CAD build for the part. Positions are in the model's coordinates, mm. Give positions to 0.01 mm unless a question says otherwise; leave off trailing zeros. Write each loop counter-clockwise with the first axis right and the second up, starting at its lowest first coordinate (ties: lowest second). Pieces come first, ordered by that corner, then holes. Notation, with made-up numbers: (24, 57.25) - (29, 57.25) arc R15 cw to (29, 68.25) - close; hole circle Ø7 at (31.5, 51.25). An arc over 180 degrees is marked (long way). Put each result on its own line as item: value. Start each with the question number.
1. Mould opens along X. For faces 1 (the cylindrical face through (-9.162, 40.474, 298.893)), 2 (the flat face through (38.538, 18, 148)), 3 (the cylindrical face through (-0.702, 40.994, 147.9)), 4 (the flat face through (-38.538, 18, 148)) say: +X half, -X half, draft (parallel to the pull), parting line (faces both ways), or undercut.
2. Drop flat-ended pins along their axis: pin 1 (3.5 mm diameter, centred on x = 0, z = 41, fed in from -Y); pin 2 (12 mm diameter, centred on x = 7, z = 53.5, fed in from -Y); pin 3 (8 mm diameter, centred on y = 36.5, z = 242.5, fed in from -X); pin 4 (3 mm diameter, centred on x = 0, z = 10, fed in from +Y). Give the stop position or say it passes through.
3. Wall check: line 1 (X direction, y = 41, z = 10); line 2 (X direction, y = 33, z = 35); line 3 (Y direction, x = 1.5, z = 92). Give the ranges that are in metal, low to high.
4. Cut at B-B on z = 134. List the corners of the cut face in (x, y), and give its area (3 significant figures).
5. Cut at C-C on x = 23.5. List the corners of the cut face in (y, z), and give its area (3 significant figures).
6. Cut at A-A on y = 26. List the corners of the cut face in (x, z), and give its area (3 significant figures).
from build123d import *

# Parameters (mm, degrees)
BOSS_EXTRU_1_DEPTH                   = 300
ENL_V_MAT_EXTRU_1_DEPTH              = 45.5
D_GAGEMENT_M21_D                     = 3.1
D_GAGEMENT_M21_CSINK_D               = 6
D_GAGEMENT_M21_CSINK_ANGLE           = 120
R_P_TITION_LIN_AIRE1_COUNT           = 2
R_P_TITION_LIN_AIRE1_PITCH           = 31
D_GAGEMENT_M41_D                     = 3.1
D_GAGEMENT_M41_DEPTH                 = 30
D_GAGEMENT_M41_CSINK_D               = 5
D_GAGEMENT_M41_CSINK_ANGLE           = 90
D_GAGEMENT_M41_TIP                   = 0.931333959
D_GAGEMENT_M41_ON_FACE_2_D           = 3.1
D_GAGEMENT_M41_ON_FACE_2_DEPTH       = 30
D_GAGEMENT_M41_ON_FACE_2_CSINK_D     = 5
D_GAGEMENT_M41_ON_FACE_2_CSINK_ANGLE = 90
D_GAGEMENT_M41_ON_FACE_2_TIP         = 0.931333959


with BuildPart() as part:
    # Esquisse1 → Boss.-Extru.1 (new body)
    with BuildSketch(Plane.XY):
        with BuildLine():
            Line((-38.538130468, 22.25), (-38.538130468, 13.993301969))
            ThreePointArc((-38.538130468, 13.993301969), (0, 41), (38.538130468, 13.993301969))
            Line((38.538130468, 13.993301969), (38.538130468, 22.25))
            ThreePointArc((38.538130468, 22.25), (0, 44.5), (-38.538130468, 22.25))
        make_face()
    extrude(amount=BOSS_EXTRU_1_DEPTH)

    # Esquisse2 → Enlèv. mat.-Extru.1 (cut, through all)
    with BuildSketch(Plane(origin=(0, 0, 0), x_dir=(1, 0, 0), z_dir=(0, 1, 0))):
        with BuildLine():
            Line((38.538130468, -261.46), (70.818354585, -261.46))
            Line((70.818354585, -261.46), (70.818354585, -316.268787276))
            Line((70.818354585, -316.268787276), (-50.118143928, -316.268787276))
            Line((-50.118143928, -316.268787276), (-50.118143928, -261.46))
            Line((-50.118143928, -261.46), (-38.538130468, -261.46))
            ThreePointArc((-38.538130468, -261.46), (0, -299.998130468), (38.538130468, -261.46))
        make_face()
    enl_v_mat_extru_1 = extrude(amount=ENL_V_MAT_EXTRU_1_DEPTH, mode=Mode.SUBTRACT)

    # Symétrie1: Enlèv. mat.-Extru.1 across plane
    add(enl_v_mat_extru_1.mirror(Plane.XY.offset(150)), mode=Mode.SUBTRACT)

    # Dégagement M21 (through all)
    with Locations(Plane(origin=(0.001869532, 44.499999961, 10), x_dir=(0.999999999, -4.2012e-05, 0), z_dir=(4.2012e-05, 0.999999999, 0))):
        with Locations((0, 0)):
            d_gagement_m21 = CounterSinkHole(D_GAGEMENT_M21_D / 2, D_GAGEMENT_M21_CSINK_D / 2, counter_sink_angle=D_GAGEMENT_M21_CSINK_ANGLE)

    # Répétition linéaire1: Dégagement M21 ×2
    with Locations(*[(0, 0, i * R_P_TITION_LIN_AIRE1_PITCH) for i in range(1, R_P_TITION_LIN_AIRE1_COUNT)]):
        add(d_gagement_m21, mode=Mode.SUBTRACT)

    # Dégagement M41
    with Locations(Plane(origin=(-12.265862334, 42.776145469, 285), x_dir=(0.961261696, 0.275637356, 0), z_dir=(-0.275637356, 0.961261696, 0))):
        with Locations((0, 0)):
            CounterSinkHole(D_GAGEMENT_M41_D / 2, D_GAGEMENT_M41_CSINK_D / 2, depth=D_GAGEMENT_M41_DEPTH, counter_sink_angle=D_GAGEMENT_M41_CSINK_ANGLE)
            with Locations((0, 0, -(D_GAGEMENT_M41_DEPTH + D_GAGEMENT_M41_TIP / 2))):  # 118° drill point
                Cone(0, D_GAGEMENT_M41_D / 2, D_GAGEMENT_M41_TIP, mode=Mode.SUBTRACT)

    # Dégagement M41 on face 2
    with Locations(Plane(origin=(12.265862334, 42.776145469, 285), x_dir=(0.961261813, -0.275636946, 0), z_dir=(0.275636946, 0.961261813, 0))):
        with Locations((0, 0)):
            CounterSinkHole(D_GAGEMENT_M41_ON_FACE_2_D / 2, D_GAGEMENT_M41_ON_FACE_2_CSINK_D / 2, depth=D_GAGEMENT_M41_ON_FACE_2_DEPTH, counter_sink_angle=D_GAGEMENT_M41_ON_FACE_2_CSINK_ANGLE)
            with Locations((0, 0, -(D_GAGEMENT_M41_ON_FACE_2_DEPTH + D_GAGEMENT_M41_ON_FACE_2_TIP / 2))):  # 118° drill point
                Cone(0, D_GAGEMENT_M41_ON_FACE_2_D / 2, D_GAGEMENT_M41_ON_FACE_2_TIP, mode=Mode.SUBTRACT)


solid = part.part
Report:
1. face 1: parting line
1. face 2: +X half
1. face 3: undercut
1. face 4: -X half
2. pin 1: stops at y = 40.96
2. pin 2: stops at y = 38.88
2. pin 3: stops at x = -30.4
2. pin 4: passes through
3. line 1: x = -17.3 to -1.55, 1.55 to 17.3
3. line 2: x = -29.85 to -24.33, 24.33 to 29.85
3. line 3: y = 40.97 to 44.47
4. outline: (-38.54, 13.99) arc R41 cw to (38.54, 13.99) - (38.54, 22.25) arc R44.5 ccw to (-38.54, 22.25) - close
4. area: 337 mm²
5. outline: (33.6, 8) - (37.79, 8) - (37.79, 292) - (33.6, 292) - close
5. area: 1,190 mm²
6. outline: (-36.11, 25.09) arc R38.54 ccw to (-31.7, 16.63) - (-31.7, 283.37) arc R38.54 ccw to (-36.11, 274.91) - close; (31.7, 16.63) arc R38.54 ccw to (36.11, 25.09) - (36.11, 274.91) arc R38.54 ccw to (31.7, 283.37) - close
6. area: 2,290 mm²
